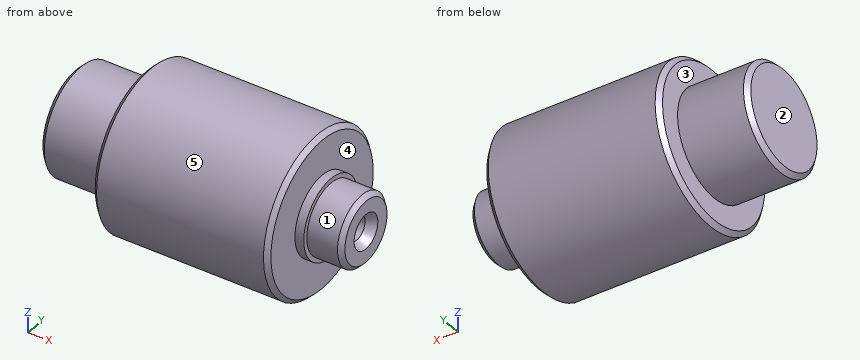
Solid Edge part; units mm, degrees
sketch "Sketch1" plane through (0, 0, 0) normal (0, -1, 0) x (1, 0, 0)
  line L0 (0, 0) -> (0, -6)
  line L1 (0, -6) -> (8, -6)
  line L2 (8, -6) -> (8, -9)
  line L3 (8, -9) -> (28, -9)
  line L4 (28, -9) -> (28, -4.5)
  line L5 (28, -4.5) -> (29, -4.5)
  line L6 (29, -4.5) -> (29, -4)
  line L7 (29, -4) -> (33, -4)
  line L8 (33, -4) -> (33, 0)
  dimension "D1" = 8
  dimension "D2" = 29
  dimension "D3" = 28
revolve "RevolvedProtrusion1" add sketch "Sketch1" angle 360 about axis through (14, 0, 0) along (-1, 0, 0)
chamfer "Chamfer1" distance 0.5 angle 45 4 edges at (0, 0, 6) (33, 0, 4) (8, 0, 9) (28, 0, 9)
hole "Hole_1" at (33, 0, 0) direction (-1, 0, 0) diameter 2.75 depth 30 tip angle 118 start chamfer 0.6 start chamfer angle 30 end chamfer 0.6 end chamfer angle 30
properties material "Polyethylene, low density"
Geometry check sheet. Reference: the model listing, model coordinates, mm. Face numbers are marked on the shaded views. A direction names the side the tool comes from. Coordinates: 2 decimals unless noted, no trailing zeros. Order: outer loops, then holes, each group sorted by start corner. A loop starts at its lowest first (then second) coordinate and runs counter-clockwise, first axis right, second up. Notation, with made-up numbers: M 4.5,28 L 60.5,28 A17 ccw 60.5,41 Z; hole C 74,63.5 d4. An arc over 180 degrees is marked long. Answer as a JSON object with one key per item and string values.
Q1. Cross-section at A-A on x = 30.5. Record the cut outline in (y, z) (3 decimals), and give its area (3 significant figures).
Results are:
{"outline": "C 0,0 d8; hole C 0,0 d2.75", "area": "44.3 mm²"}
Q2. Tool access check on the marked faces 3, 4 and 5. Record the directions out of +Z, -Z, +X, -X, +Y, -Y that give a thin tool (end or side, any length) a straight path to the whole face; none if there is none.
Results are:
{"face 3": "-X", "face 4": "+X", "face 5": "+X, -X"}
Q3. Depth check by flat-ended pin: pin 1 Ø1 at (x, y) = (25, -1.5) entering from +Z; pin 2 Ø4 at (x, y) = (19.5, 3) entering from -Z; pin 3 Ø1 at (y, z) = (4.5, 4.5) entering from +X. Enter the tip coordinate at first touch or a pass-through.
Results are:
{"pin 1": "stops at z = 8.94", "pin 2": "stops at z = -8.94", "pin 3": "stops at x = 28"}
Q4. Cross-section at B-B on x = 23. Record the cut outline in (y, z) (3 decimals), and give its area (3 significant figures).
Results are:
{"outline": "C 0,0 d18; hole C 0,0 d2.75", "area": "249 mm²"}
Q5. Scan lines: line 1 (Z direction, x = 14.5, y = 0) (3 decimals); line 2 (X direction, y = -4.75, z = -0.5). Record each from-to range of solid material in increasing order.
Results are:
{"line 1": "z = -9 to -1.375, 1.375 to 9", "line 2": "x = 0 to 28"}
Q6. Release check for a two-part mould opening along Z. For the marked faces 1 and 2 record: released by +Z, released by -Z, zero draft, split by the parting line, or undercut.
Results are:
{"face 1": "split by the parting line", "face 2": "zero draft"}
